Could you check a few things on this model? Use its own coordinates, in mm. Give positions to 0.01 mm unless a question says otherwise; leave off trailing zeros. Order: outer loops, then holes, each group sorted by start corner. A loop starts at its lowest first (then second) coordinate and runs counter-clockwise, first axis right, second up.
(1) If I drill on probe 1 along X at (y, z) = (-2.75, 5); probe 2 along Z at (x, y) = (-6.25, -4.5); probe 3 along Z at (x, y) = (4.75, -3.5), over which ranges is the centre line in solid material (lowest first)?
(2) Imagine slicing it at B-B, the plane y = -2.5. Write out the boundary of the cut face in (x, z), then the cut area to 3 significant figures.
(3) If we mould it in two halves opening along X, with no side actions, what happens to faces 1 (the flat face through (-12, -4, 0)), 2 (the flat face through (6.084, -4.056, -10.344)), 3 (the cylindrical face through (-0.936, -4.045, 7.127))? For each: released by +X, released by -X, zero draft, split by the parting line, or undercut.
(4) Imagine slicing it at A-A, the plane z = 0. Write out the boundary of the cut face in (x, y), then the cut area to 3 significant figures.
Autodesk Inventor part; units mm, degrees
ref_plane "2CYL_XY" through (0, -4, 0) normal (0, 1, 0) x (1, 0, 0)
ref_plane "2CYL_YZ" through (0, -4, 0) normal (1, 0, 0) x (0, 0, -1)
ref_plane "2CYL_ZX" through (0, -4, 0) normal (0, 0, -1) x (0, 1, 0)
sketch "Sketch_1" plane through (0, 0, 0) normal (0, 0, 1) x (1, 0, 0)
  line L0 (0, -8) -> (0, 0)
  line L1 (0, 0) -> (11.95, 0)
  line L2 (11.95, 0) -> (26.8782, -4)
  line L3 (26.8782, -4) -> (11.95, -8)
  line L4 (11.95, -8) -> (0, -8)
  line L5 (0, -8) -> (0, 0)
revolve "Revolution1" add sketch "Sketch_1" angle 360 about axis through (0, -8, 0) along (0, 1, 0)
sketch "Sketch_2" plane through (0, 0, 0) normal (0, 1, 0) x (-1, 0, 0)
  line L0 (48, -48) -> (48, 48)
  line L1 (48, 48) -> (-48, 48)
  line L2 (-48, 48) -> (-48, -48)
  line L3 (-48, -48) -> (48, -48)
  line L4 (12, 6.9282) -> (0, 13.8564)
  line L5 (0, 13.8564) -> (-12, 6.9282)
  line L6 (-12, 6.9282) -> (-12, -6.9282)
  line L7 (-12, -6.9282) -> (0, -13.8564)
  line L8 (0, -13.8564) -> (12, -6.9282)
  line L9 (12, -6.9282) -> (12, 6.9282)
extrude "Extrusion1" cut sketch "Sketch_2" along normal mid plane 18
sketch "Sketch_3" plane through (0, 0, 0) normal (0, 0, 1) x (1, 0, 0)
  line L0 (0, -8) -> (0, 0)
  line L1 (0, 0) -> (8, 0)
  line L2 (8, 0) -> (7.188, -0.812)
  line L3 (7.188, -0.812) -> (7.188, -7.188)
  line L4 (7.188, -7.188) -> (8, -8)
  line L5 (8, -8) -> (0, -8)
  line L6 (0, -8) -> (0, 0)
revolve "Revolution2" cut sketch "Sketch_3" angle 360 about axis through (0, -8, 0) along (0, -1, 0)
thread "Thread1"
ref_plane "2CYL_XY" through (0, -4, 0) normal (0, 1, 0) x (1, 0, 0)
ref_plane "2CYL_YZ" through (0, -4, 0) normal (1, 0, 0) x (0, 0, -1)
ref_plane "2CYL_ZX" through (0, -4, 0) normal (0, 0, -1) x (0, 1, 0)
ref_plane "din439b_punkt_XY" through (0, 0, 0) normal (0, 1, 0) x (1, 0, 0)
ref_plane "din439b_punkt_YZ" through (0, 0, 0) normal (1, 0, 0) x (0, 0, -1)
ref_plane "din439b_punkt_ZX" through (0, 0, 0) normal (0, 0, -1) x (0, 1, 0)
properties part number "DIN-439-B - M16x1.5(F)"
Answer block:
1. probe 1: x = -12 to -5.16, 5.16 to 12
1. probe 2: z = -10.25 to -3.55, 3.55 to 10.25
1. probe 3: z = -11.11 to -5.39, 5.39 to 11.11
2. outline: (-12, -6.93) - (0, -13.86) - (12, -6.93) - (12, 6.93) - (0, 13.86) - (-12, 6.93) - close; hole circle Ø14.38 at (0, 0)
2. area: 337 mm2
3. face 1: released by -X
3. face 2: released by +X
3. face 3: undercut
4. outline: (-12, -7.99) - (-11.95, -8) - (-8, -8) - (-7.19, -7.19) - (-7.19, -0.81) - (-8, 0) - (-11.95, 0) - (-12, -0.01) - close; (7.19, -7.19) - (8, -8) - (11.95, -8) - (12, -7.99) - (12, -0.01) - (11.95, 0) - (8, 0) - (7.19, -0.81) - close
4. area: 75.7 mm2
